Geometry check sheet. Reference: the model listing, model coordinates, mm. A direction names the side the tool comes from. Give positions to 0.01 mm unless a question says otherwise; leave off trailing zeros. Write each loop counter-clockwise with the first axis right and the second up, starting at its lowest first coordinate (ties: lowest second). Pieces come first, ordered by that corner, then holes. Notation, with made-up numbers: M 71,-10.75 L 121,-10.75 A9 cw 121,3.25 Z; hole C -0.5,65.25 d1. An arc over 180 degrees is marked long. Write each question's results on one line, items separated by ' | '.
```python
from build123d import *

# Parameters (mm, degrees)
BOSS_EXTRUDE1_DEPTH     = 17
CUT_EXTRUDE1_DEPTH      = 2.5
SKETCH5_W               = 2.5
SKETCH5_H               = 19.830535888
CUT_EXTRUDE2_DEPTH      = 2.5
EXTRUDE_THIN1_DEPTH     = 4.5
SKETCH8_R               = 8.5
CUT_EXTRUDE4_DEPTH      = 6.5
SKETCH9_R               = 5
CUT_EXTRUDE5_DEPTH      = 27.5
CUT_EXTRUDE6_DEPTH      = 0.5
CUT_EXTRUDE6_DEPTH_BACK = 1
SKETCH10_R              = 6
CUT_EXTRUDE7_START      = -12.5
SKETCH14_R              = 9.571158882
CUT_EXTRUDE7_DEPTH      = 12.5
SKETCH12_R              = 10.071158882
SKETCH12_R_2            = 8.071158882
CUT_EXTRUDE_THIN1_DEPTH = 5
SKETCH15_W              = 2.588485832
SKETCH15_H              = 17.190343429
CUT_EXTRUDE8_DEPTH      = 31.5


with BuildPart() as part:
    # Sketch1 → Boss-Extrude1 (new body)
    with BuildSketch(Plane.XY):
        with BuildLine():
            Line((17.875866164, 9.915267944), (17.875866164, -9.915267944))
            ThreePointArc((17.875866164, -9.915267944), (-16.242631254, 0), (17.875866164, 9.915267944))
        make_face()
    extrude(amount=BOSS_EXTRUDE1_DEPTH)

    # Sketch4 → Cut-Extrude1 (cut)
    with BuildSketch(Plane.XY.offset(17)):
        with BuildLine():
            Line((16.875866164, -9.620266797), (16.875866164, 9.620266797))
            ThreePointArc((16.875866164, 9.620266797), (-15.242631254, 0), (16.875866164, -9.620266797))
        make_face()
    extrude(amount=-CUT_EXTRUDE1_DEPTH, mode=Mode.SUBTRACT)

    # Sketch5 → Cut-Extrude2 (cut)
    with BuildSketch(Plane(origin=(17.875866164, 0, 0), x_dir=(0, 0, -1), z_dir=(1, 0, 0))):
        with Locations((-15.75, 0)):
            Rectangle(SKETCH5_W, SKETCH5_H)
    extrude(amount=-CUT_EXTRUDE2_DEPTH, mode=Mode.SUBTRACT)

    # Sketch6 → Extrude-Thin1 (add)
    with BuildSketch(Plane.XY.offset(14.5)):
        with BuildLine():
            ThreePointArc((15.440925449, 7.665267944), (17.39404784, 0), (15.440925449, -7.665267944))
            ThreePointArc((15.440925449, -7.665267944), (-12.992631254, 0), (15.440925449, 7.665267944))
        make_face()
        with BuildLine():
            ThreePointArc((14.787338867, 7.297249398), (16.64404784, 0), (14.787338867, -7.297249398))
            ThreePointArc((14.787338867, -7.297249398), (-12.242631254, 0), (14.787338867, 7.297249398))
        make_face(mode=Mode.SUBTRACT)
    extrude(amount=EXTRUDE_THIN1_DEPTH)

    # Sketch8 → Cut-Extrude4 (cut)
    with BuildSketch(Plane(origin=(0, 0, 0), x_dir=(-1, 0, 0), z_dir=(0, 0, -1))):
        with Locations((-2.257368746, 0)):
            Circle(SKETCH8_R)
    extrude(amount=-CUT_EXTRUDE4_DEPTH, mode=Mode.SUBTRACT)

    # Sketch9 → Cut-Extrude5 (cut)
    with BuildSketch(Plane(origin=(0, 0, 6.5), x_dir=(-1, 0, 0), z_dir=(0, 0, -1))):
        with Locations((-2.257368746, 0)):
            Circle(SKETCH9_R)
    extrude(amount=-CUT_EXTRUDE5_DEPTH, mode=Mode.SUBTRACT)

    # Sketch10 → Cut-Extrude6 (cut, two sides: drawn at the far end of the back side and taken through both)
    with BuildSketch(Plane(origin=(0, 0, 6.5), x_dir=(-1, 0, 0), z_dir=(0, 0, -1)).offset(-CUT_EXTRUDE6_DEPTH_BACK)):
        with Locations((-2.257368746, 0)):
            Circle(SKETCH10_R)
    extrude(amount=CUT_EXTRUDE6_DEPTH + CUT_EXTRUDE6_DEPTH_BACK, mode=Mode.SUBTRACT)

    # Sketch14 → Cut-Extrude7 (cut)
    with BuildSketch(Plane.XY.offset(14.5).offset(CUT_EXTRUDE7_START)):
        with BuildLine():
            ThreePointArc((14.787338867, 7.297249398), (-12.242631254, 0), (14.787338867, -7.297249398))
            ThreePointArc((14.787338867, -7.297249398), (16.64404784, 0), (14.787338867, 7.297249398))
        make_face()
        with Locations((2.257368746, 0)):
            Circle(SKETCH14_R, mode=Mode.SUBTRACT)
    extrude(amount=CUT_EXTRUDE7_DEPTH, mode=Mode.SUBTRACT)

    # Sketch12 → Cut-Extrude-Thin1 (cut)
    with BuildSketch(Plane.XY.offset(14.5)):
        with Locations((2.257368746, 0)):
            Circle(SKETCH12_R)
        with Locations((2.257368746, 0)):
            Circle(SKETCH12_R_2, mode=Mode.SUBTRACT)
    extrude(amount=-CUT_EXTRUDE_THIN1_DEPTH, mode=Mode.SUBTRACT)

    # Sketch15 → Cut-Extrude8 (cut)
    with BuildSketch(Plane.XY):
        with Locations((-16.39432519, -0.486978568)):
            Rectangle(SKETCH15_W, SKETCH15_H)
    extrude(amount=CUT_EXTRUDE8_DEPTH, mode=Mode.SUBTRACT)


solid = part.part
```
Q1. Section check C-C (z = 4.5). Enter the section's corners in (x, y).
Answer key:
outline: M -15.1,-6.4 A18.5 ccw 17.88,-9.92 L 17.88,9.92 A18.5 ccw -15.1,6.4 Z; C 2.26,0 d19.14; hole C 2.26,0 d17; hole M 14.79,-7.3 A15.27 ccw 14.79,7.3 A14.5 ccw long Z
Q2. Material ranges on probe 1 along X at (y, z) = (-0.5, 3.25); probe 2 along X at (y, z) = (-4, 8.5); probe 3 along Z at (x, y) = (14.5, -7), recorded low to high. Write a range as [from, to].
Answer key:
probe 1: x = [-15.1, -12.23], [-7.3, -6.23], [10.74, 11.82], [16.64, 17.88] | probe 2: x = [-15.1, -11.68], [-6.44, -0.74], [5.26, 10.95], [16.11, 17.88] | probe 3: z = [0, 2]
Q3. Section check A-A (z = 11.5). Enter the section's corners in (x, y), then the cut area to 3 significant figures.
Answer key:
outline: M -15.1,-6.4 A18.5 ccw 17.88,-9.92 L 17.88,9.92 A18.5 ccw -15.1,6.4 Z; C 2.26,0 d16.14; hole C 2.26,0 d10; hole M 14.79,-7.3 A15.27 ccw 14.79,7.3 A14.5 ccw long Z | area: 493 mm2
Q4. Depth check by flat-ended pin: P1, Ø3, axis at y = -9.5, z = 17, coming from the -X side; P2, Ø4, axis at x = 1.5, y = -1.5, coming from the -Z side; P3, Ø5, axis at x = -2, y = 9, coming from the +Z side; P4, Ø3, axis at x = -10, z = 11, coming from the -Y side. Enter the tip coordinate at first touch or a pass-through.
Answer key:
P1: stops at x = -14.42 | P2: passes through | P3: stops at z = 14.5 | P4: stops at y = -15.05
Q5. Access from +Z, -Z, +X, -X, +Y, -Y to the whole of each face (thin tool, end or side, straight path). Record for faces 4 (the face through (0, 18, 17)), 5 (the face through (-2.14, -16.94, 15.77)), 6 (the face through (-3.466, 1.802, 7.007)), 7 (the face through (17.394, 0.112, 16.718)).
Answer key:
face 4: +Z, +Y | face 5: +Z | face 6: -Z | face 7: +Z, +X
Q6. Release check for a two-part mould opening along Y. For faces 1 (the face through (17.876, 0, 7)), 2 (the face through (0.583, -18.424, 8.381)), 3 (the face through (17, -9.915, 16)) record: released by +Y, released by -Y, zero draft, split by the parting line, or undercut.
Answer key:
face 1: zero draft | face 2: released by -Y | face 3: undercut
Q7. Section check D-D (x = 9.5). Enter the section's corners in (y, z).
Answer key:
outline: M -17.02,0 L -4.45,0 L -4.45,6.5 L 4.45,6.5 L 4.45,0 L 17.02,0 L 17.02,17 L 15.93,17 L 15.93,14.5 L 13.42,14.5 L 13.42,19 L 12.56,19 L 12.56,2 L 6.26,2 L 6.26,9.5 L 3.56,9.5 L 3.56,14.5 L -3.56,14.5 L -3.56,9.5 L -6.26,9.5 L -6.26,2 L -12.56,2 L -12.56,19 L -13.42,19 L -13.42,14.5 L -15.93,14.5 L -15.93,17 L -17.02,17 Z
